from build123d import *

# Parameters (mm, degrees)
SKETCH_1_R      = 1.5
EXTRUDE_1_DEPTH = 3
CHAMFER_1_SIZE  = 1.7


with BuildPart() as part:
    # Эскиз1 → Бобышка-Вытянуть1 (new body)
    with BuildSketch(Plane.XY):
        with BuildLine():
            Line((38.4, -38.5), (38.4, 38.5))
            ThreePointArc((38.4, 38.5), (37.111269837, 41.611269837), (34, 42.9))
            Line((34, 42.9), (-34, 42.9))
            ThreePointArc((-34, 42.9), (-37.111269837, 41.611269837), (-38.4, 38.5))
            Line((-38.4, 38.5), (-38.4, -38.5))
            ThreePointArc((-38.4, -38.5), (-37.111269837, -41.611269837), (-34, -42.9))
            Line((-34, -42.9), (34, -42.9))
            ThreePointArc((34, -42.9), (37.111269837, -41.611269837), (38.4, -38.5))
        make_face()
        with Locations((34, -38.5)):
            Circle(SKETCH_1_R, mode=Mode.SUBTRACT)
        with Locations(Location((-34, -38.5, 0), (0, 0, 180))):
            Circle(SKETCH_1_R, mode=Mode.SUBTRACT)
        with Locations(Location((34, 38.5, 0), (0, 0, 180))):
            Circle(SKETCH_1_R, mode=Mode.SUBTRACT)
        with Locations((-34, 38.5)):
            Circle(SKETCH_1_R, mode=Mode.SUBTRACT)
    extrude(amount=EXTRUDE_1_DEPTH)

    # Фаска1
    chamfer_1_edges = [part.edges().sort_by_distance(p)[0] for p in [
        (32.5, -38.5, 3),
        (-32.5, -38.5, 3),
        (35.5, 38.5, 3),
        (-35.5, 38.5, 3),
    ]]
    chamfer(chamfer_1_edges, length=CHAMFER_1_SIZE)


solid = part.part
Design review of the part built by this model. Coordinates are the model's own, in mm. Give positions to 0.01 mm unless a question says otherwise; leave off trailing zeros. Order: outer loops, then holes, each group sorted by start corner. A loop starts at its lowest first (then second) coordinate and runs counter-clockwise, first axis right, second up. Notation, with made-up numbers: (13.25, -24) - (67.25, -24) arc R23 ccw to (67.25, 10) - close; hole circle Ø4 at (-31, 36). An arc over 180 degrees is marked (long way). Use CSV: the item, a comma, the result in double quotes. Start each with the question number.
Q1. Draft analysis for pull direction X (two halves, no side actions). For faces 1 (the face through (-1, 1, 3)), 2 (the face through (-35.2, 37.6, 0.6)), 3 (the face through (-37.145, -41.577, 1.479)), state which applies: pulls with the +X half, pulls with the -X half, needs draft (parallel to the pull), parting line crosses it, or undercut.
Q2. For line 1 (Y direction, x = -34, z = 0.45), list the stretches that pass through material, from the lowest coordinate up.
Q3. Take a section at A-A (z = 2.4). State the section outline as (x, y) points, and give its area (3 significant figures).
Q4. For P1, Ø2.5, axis at x = 34, y = -38.5, coming from the -Z side; P2, Ø5, axis at x = -34, y = -38.5, coming from the +Z side, all flat-tipped, find the tip position at first contact; note any pin that passes through.
Calculated:
1,face 1,"needs draft"
1,face 2,"undercut"
1,face 3,"pulls with the -X half"
2,line 1,"y = -42.9 to -40, -37 to 37, 40 to 42.9"
3,outline,"(-38.4, -38.5) arc R4.4 ccw to (-34, -42.9) - (34, -42.9) arc R4.4 ccw to (38.4, -38.5) - (38.4, 38.5) arc R4.4 ccw to (34, 42.9) - (-34, 42.9) arc R4.4 ccw to (-38.4, 38.5) - close; hole circle Ø5.2 at (-34, -38.5); hole circle Ø5.2 at (-34, 38.5); hole circle Ø5.2 at (34, -38.5); hole circle Ø5.2 at (34, 38.5)"
3,area,"6,490 mm²"
4,P1,"passes through"
4,P2,"stops at z = 2.3"
